Autodesk Inventor part; units mm, degrees
ref_plane "Work Plane1" through (0, 6.35, 0) normal (0, 1, 0) x (1, 0, 0)
ref_plane "YZ Plane" through (0, 0, 0) normal (1, 0, 0) x (0, 1, 0)
ref_plane "XZ Plane" through (0, 0, 0) normal (0, 1, 0) x (-1, 0, 0)
sketch "Sketch1" plane through (0, 0, 0) normal (0, 1, 0) x (-1, 0, 0)
  circle A0 centre (0, 0) radius 3.302
  line L0 (0, 0) -> (3.302, 0)
  arc A1 (6.35, 0) -> (4.8481, 14.975) centre (-69.0563, 0) ccw
  circle A2 centre (-69.0563, 0) radius 69.0563 construction
  circle A3 centre (-0.5908, 9.0136) radius 1.5875
  line L1 (-0.5908, 9.0136) -> (-69.0563, 0) construction
  circle A4 centre (-0.5908, 9.0136) radius 4.7625
  line L2 (9.5157, 15.9208) -> (-1.5366, 13.6813)
  arc A5 (11.1125, 0) -> (9.5157, 15.9208) centre (-69.0563, 0) ccw
  arc A6 (-4.7625, 0) -> (-5.3125, 8.392) centre (-69.0563, 0) ccw
  line L3 (0, 0) -> (-69.0563, 0) construction
  arc A7 (4.8481, -14.975) -> (6.35, 0) centre (-69.0563, 0) ccw
  circle A8 centre (-0.5908, -9.0136) radius 1.5875
  circle A9 centre (-0.5908, -9.0136) radius 4.7625
  line L4 (9.5157, -15.9208) -> (-1.5366, -13.6813)
  arc A10 (9.5157, -15.9208) -> (11.1125, 0) centre (-69.0563, 0) ccw
  arc A11 (-5.3125, -8.392) -> (-4.7625, 0) centre (-69.0563, 0) ccw
  point P0 (4.8277, -15.4708)
  dimension "d0" = 6.604
  dimension "d1" = 6.35
  dimension "d2" = 75.4062
  dimension "d3" = 3.175
  dimension "d6" = 9.525
  dimension "d7" = 4.7625
  dimension "d8" = 7.5
  dimension "d14" = 138.1125
extrude "Extrusion1" add sketch "Sketch1" along normal blind 12.7 contours A7 L4 A9 A11 A6 A4 L2 A1 | A4 | A9
extrude "Extrusion2" add sketch "Sketch1" against normal blind 3.175
ref_plane "Work Plane1" through (0, 6.35, 0) normal (0, 1, 0) x (1, 0, 0)
mirror "Mirror1" about plane through (0, 6.35, 0) normal (0, 1, 0) of "Extrusion2"
fillet "Fillet1" radius 3.175 6 edges at (-9.5157, 14.2875, 15.9208) (-9.5157, 14.2875, -15.9208) (-9.5157, -1.5875, -15.9208) (-9.5157, -1.5875, 15.9208) (-4.8481, 6.35, 14.975) (-4.8481, 6.35, -14.975)
properties part number "Braces"
Verification items for the finished model (mm, model axes). A direction names the side the tool comes from. Coordinates: 2 decimals unless noted, no trailing zeros. Order: outer loops, then holes, each group sorted by start corner. A loop starts at its lowest first (then second) coordinate and runs counter-clockwise, first axis right, second up. Notation, with made-up numbers: M -38.5,85.25 L 18.5,85.25 A21 cw 18.5,104.25 Z; hole C 42,-1.5 d8. An arc over 180 degrees is marked long. One line per item, written item: value. Start each with the question number.
Item 1: Sectioned sample at A-A on x = 1. Record the cut outline in (y, z) (3 decimals), then the cut area to 3 significant figures.
Item 2: Sectioned sample at C-C on y = 9.5. Give the number of separate pieces and of enclosed holes in the cut face, then the cut area to 3 significant figures.
Item 3: Sectioned sample at D-D on x = -6. Record the cut outline in (y, z) (3 decimals), then the cut area to 3 significant figures.
Item 4: Access from +Z, -Z, +X, -X, +Y, -Y to the whole of each face (thin tool, end or side, straight path). Record for faces 4 (the cylindrical face through (-6.114, 6.261, 5.956)), 5 (the cylindrical face through (4.896, 6.217, -4.146)), 6 (the cylindrical face through (-0.142, 6.217, 10.422)), 7 (the cylindrical face through (-10.853, 14.265, 6.442)), 8 (the cylindrical face through (-6.127, 6.261, -5.792)).
Item 5: Depth check by flat-ended pin: P1, Ø1.5, axis at x = -4, y = 13, coming from the +Z side; P2, Ø2, axis at y = 4.5, z = 11.5, coming from the -X side; P3, Ø1, axis at y = 3.5, z = -1, coming from the -X side. Enter the tip coordinate at first touch or a pass-through.
Item 6: Mould release check, pull along Z, two halves, no side actions. Record for faces 1 (the cylindrical face through (-4.081, 6.439, -13.846)), 2 (the cylindrical face through (0.797, 6.217, -10.588)), 3 (the cylindrical face through (-8.749, -1.61, 14.795)): pulls with the +Z half, pulls with the -Z half, needs draft (parallel to the pull), parting line crosses it, or undercut.
Item 7: Thickness scan on probe 1 along Z at (x, y) = (2, 6); probe 2 along Z at (x, y) = (-0.5, 5); probe 3 along Y at (x, z) = (-6.5, 6) (3 decimals). Record the ranges inside material, lowest first.
Item 8: Sectioned sample at B-B on z = 0.5. Record the cut outline in (x, y) (3 decimals).
Calculated:
1. outline: M -3.175,-13.79 L 15.875,-13.79 L 15.875,-10.547 L -3.175,-10.547 Z; M -3.175,-7.48 L 15.875,-7.48 L 15.875,-3.147 L -3.175,-3.147 Z; M -3.175,3.147 L 15.875,3.147 L 15.875,7.48 L -3.175,7.48 Z; M -3.175,10.547 L 15.875,10.547 L 15.875,13.79 L -3.175,13.79 Z
1. area: 289 mm^2
2. separate pieces: 1
2. enclosed holes: 3
2. area: 247 mm^2
3. outline: M -3.175,-15.208 L 0,-15.208 L 0,-7.257 L 12.7,-7.257 L 12.7,-15.208 L 15.875,-15.208 L 15.875,15.208 L 12.7,15.208 L 12.7,7.257 L 0,7.257 L 0,15.208 L -3.175,15.208 Z
3. area: 377 mm^2
4. face 4: +Z, -X
4. face 5: +X, +Y, -Y
4. face 6: +Y, -Y
4. face 7: +Z, -X, +Y, -Y
4. face 8: -Z, -X
5. P1: z = 14.96
5. P2: x = -5.62
5. P3: x = -6.35
6. face 1: pulls with the -Z half
6. face 2: undercut
6. face 3: pulls with the +Z half
7. probe 1: -13.56 to -9.74, -8.28 to -2.63, 2.63 to 8.28, 9.74 to 13.56
7. probe 2: -14.09 to -10.17, -7.86 to -3.26, 3.26 to 7.86, 10.17 to 14.09
7. probe 3: -3.175 to 0, 12.7 to 15.875
8. outline: M -11.111,-3.175 L -3.264,-3.175 L -3.264,15.875 L -11.111,15.875 L -11.111,12.7 L -6.348,12.7 L -6.348,0 L -11.111,0 Z; M 3.264,-3.175 L 4.764,-3.175 L 4.764,15.875 L 3.264,15.875 Z
